from build123d import *

# Parameters (mm, degrees)
F0_R     = 6
F0_R_2   = 4.25
F1_DEPTH = 13
F2_W     = 13
F2_H     = 2.833082
F2_H_2   = 2.897769
F3_DEPTH = 34.5
F4_R     = 4.25
F5_DEPTH = 13.001
F6_R     = 1.75
F7_DEPTH = 8.930851


with BuildPart() as f1:
    # F0 (on Front) → F1 (new body)
    with BuildSketch(Plane.XZ):
        Circle(F0_R)
        Circle(F0_R_2, mode=Mode.SUBTRACT)
    extrude(amount=-F1_DEPTH)

    # F2 (on Right) → F3 (join)
    with BuildSketch(Plane.YZ):
        with Locations((6.5, 3.016541)):
            Rectangle(F2_W, F2_H)
        with Locations((6.5, -3.048884)):
            Rectangle(F2_W, F2_H_2)
    extrude(amount=F3_DEPTH)

    # F4 (on face) → F5 (cut, through all)
    with BuildSketch(Plane(origin=(0, 13, 0), x_dir=(-1, 0, 0), z_dir=(0, 1, 0))):
        Circle(F4_R)
    extrude(amount=-F5_DEPTH, mode=Mode.SUBTRACT)

    # F6 (on face) → F7 (cut, through all)
    with BuildSketch(Plane.XY.offset(4.433082)):
        with Locations((14.5, 6.5)):
            Circle(F6_R)
        with Locations((24.5, 6.5)):
            Circle(F6_R)
    extrude(amount=-F7_DEPTH, mode=Mode.SUBTRACT)


solid = f1.part
For this review, take the finished solid that the model builds, in its own axes (mm). A direction names the side the tool comes from. Round coordinates to 2 decimals unless told otherwise and drop trailing zeros. Write each loop counter-clockwise with the first axis right and the second up, starting at its lowest first coordinate (ties: lowest second). Pieces come first, ordered by that corner, then holes. Notation, with made-up numbers: M 80,-29 L 104,-29 A17 ccw 104,-9 Z; hole C 23.25,89.5 d7. An arc over 180 degrees is marked long. Write item = value, one per line. Start each with the question number.
(1) Clearance check with flat-ended pins moving along their axes: pin 1 Ø4.5 at (x, y) = (24.5, 6.5) entering from -Z; pin 2 Ø1.5 at (y, z) = (9.5, -4) entering from -X. State where each tip first meets the part, or that it passes through.
(2) For line 1 along Z through (x, y) = (21, 1.5); line 2 along Y through (x, z) = (14.5, -3.6); line 3 along X through (y, z) = (9, 2.5), list the stretches that pass through material, from the lowest coordinate up.
(3) We need section B-B (z = 2.5). Give the boundary of the cut face in (x, y).
(4) We need section C-C (y = 11.75). Give the boundary of the cut face in (x, z).
(5) For faces 1 (the face through (1.628, 6.409, 3.926)), 2 (the face through (20, 6, -1.6)), 3 (the face through (19, 6, 4.433)), list the 3-axis set-ups (+Z, -Z, +X, -X, +Y, -Y) from which the entire face can be reached by the end or side of a thin tool; tool diameter is ignored.
(6) The part is to be moulded in two halves that separate along X. For faces 4 (the face through (23.11, 5.44, 3.04)), 5 (the face through (34.5, 6, -3)), 6 (the face through (19, 6, -4.498)), say which applies: +X half, -X half, draft (parallel to the pull), parting line (faces both ways), or undercut.
(7) We need section D-D (x = 14.5). Give the boundary of the cut face in (y, z), then the cut area to 3 significant figures.
(8) We need section A-A (x = 0). Give the boundary of the cut face in (y, z).
Results found:
q1.pin_1 = -4.5
q1.pin_2 = -5.04
q2.line_1 = -4.5 to -1.6, 1.6 to 4.43
q2.line_2 = 0 to 4.75, 8.25 to 13
q2.line_3 = -5.45 to -3.44, 3.44 to 34.5
q3.outline = M -5.45,0 L -3.44,0 L -3.44,13 L -5.45,13 Z; M 3.44,0 L 34.5,0 L 34.5,13 L 3.44,13 Z; hole C 14.5,6.5 d3.5; hole C 24.5,6.5 d3.5
q4.outline = M 3.97,-4.5 L 34.5,-4.5 L 34.5,-1.6 L 5.78,-1.6 A6 ccw 5.78,1.6 L 34.5,1.6 L 34.5,4.43 L 4.04,4.43 A6 ccw long Z; hole C 0,0 d8.5
q5.face_1 = +Y, -Y
q5.face_2 = +X, +Y, -Y
q5.face_3 = +Z, +X, +Y, -Y
q6.face_4 = undercut
q6.face_5 = +X half
q6.face_6 = draft
q7.outline = M 0,-4.5 L 4.75,-4.5 L 4.75,-1.6 L 0,-1.6 Z; M 0,1.6 L 4.75,1.6 L 4.75,4.43 L 0,4.43 Z; M 8.25,-4.5 L 13,-4.5 L 13,-1.6 L 8.25,-1.6 Z; M 8.25,1.6 L 13,1.6 L 13,4.43 L 8.25,4.43 Z
q7.area = 54.4 mm²
q8.outline = M 0,-6 L 13,-6 L 13,-4.25 L 0,-4.25 Z; M 0,4.25 L 13,4.25 L 13,6 L 0,6 Z
